Geometry check sheet. Reference: the model listing, model coordinates, mm. Coordinates: 2 decimals unless noted, no trailing zeros. Write each loop counter-clockwise with the first axis right and the second up, starting at its lowest first coordinate (ties: lowest second). Pieces come first, ordered by that corner, then holes. Notation, with made-up numbers: (73.25, -14) -> (91.25, -14) arc R18 cw to (91.25, 13) -> close; hole circle Ø4 at (82.25, 38). An arc over 180 degrees is marked (long way). Put each result on its own line as item: value. Start each with the question number.
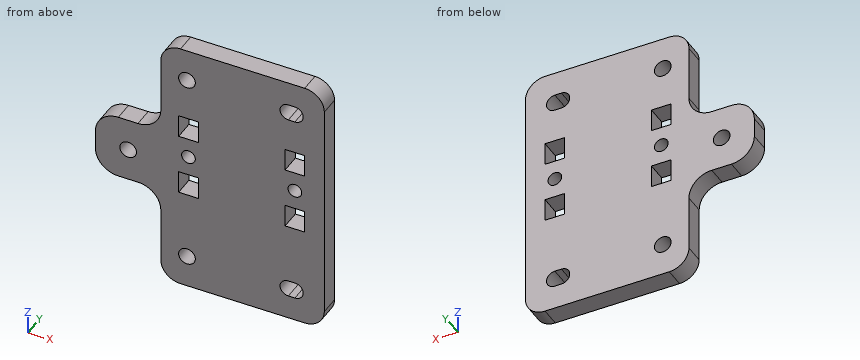
from build123d import *

# Parameters (mm, degrees)
SKETCH_1_R           = 2.55
EXTRUDE_1_DEPTH      = 6
SKETCH_2_R           = 2.55
CUT_EXTRUDE_1_DEPTH  = 7
SKETCH_3_R           = 2.1
SKETCH_3_W           = 7
SKETCH_3_H           = 6
CUT_EXTRUDE_11_DEPTH = 7
SKETCH_31_R          = 2.1
SKETCH_31_W          = 7
SKETCH_31_H          = 6
CUT_EXTRUDE_12_DEPTH = 7


with BuildPart() as part:
    # Эскиз1 → Бобышка-Вытянуть1 (new body)
    with BuildSketch(Plane(origin=(0, 0, 0), x_dir=(1, 0, 0), z_dir=(0, 1, 0))):
        with BuildLine():
            Line((-32, -10), (-38, -10))
            ThreePointArc((-38, -10), (-42.949747468, -7.949747468), (-45, -3))
            Line((-45, -3), (-45, 3))
            ThreePointArc((-45, 3), (-42.949747468, 7.949747468), (-38, 10))
            Line((-38, 10), (-32, 10))
            ThreePointArc((-32, 10), (-27.050252532, 12.050252532), (-25, 17))
            Line((-25, 17), (-25, 34))
            ThreePointArc((-25, 34), (-23.242640687, 38.242640687), (-19, 40))
            Line((-19, 40), (19, 40))
            ThreePointArc((19, 40), (23.242640687, 38.242640687), (25, 34))
            Line((25, 34), (25, -34))
            ThreePointArc((25, -34), (23.242640687, -38.242640687), (19, -40))
            Line((19, -40), (-19, -40))
            ThreePointArc((-19, -40), (-23.242640687, -38.242640687), (-25, -34))
            Line((-25, -34), (-25, -17))
            ThreePointArc((-25, -17), (-27.050252532, -12.050252532), (-32, -10))
        make_face()
        with Locations((-35, 0)):
            Circle(SKETCH_1_R, mode=Mode.SUBTRACT)
    extrude(amount=EXTRUDE_1_DEPTH)

    # Эскиз2 → Вырез-Вытянуть1 (cut, through all)
    with BuildSketch(Plane.XZ):
        with Locations((-17, -30)):
            Circle(SKETCH_2_R)
        with Locations((-17, 30)):
            Circle(SKETCH_2_R)
        with BuildLine():
            Line((16, -32.55), (14, -32.55))
            ThreePointArc((14, -32.55), (11.45, -30), (14, -27.45))
            Line((14, -27.45), (16, -27.45))
            ThreePointArc((16, -27.45), (18.55, -30), (16, -32.55))
        make_face()
        with BuildLine():
            Line((16, 32.55), (14, 32.55))
            ThreePointArc((14, 32.55), (11.45, 30), (14, 27.45))
            Line((14, 27.45), (16, 27.45))
            ThreePointArc((16, 27.45), (18.55, 30), (16, 32.55))
        make_face()
    extrude(amount=-CUT_EXTRUDE_1_DEPTH, mode=Mode.SUBTRACT)

    # Эскиз3 → Вырез-Вытянуть11 (cut, through all)
    with BuildSketch(Plane(origin=(-31, 0, 4), x_dir=(0, 0, -1), z_dir=(0, -1, 0))):
        with Locations((0, 47)):
            Circle(SKETCH_3_R)
        with Locations((9.531849908, 47)):
            Rectangle(SKETCH_3_W, SKETCH_3_H)
        with Locations((-9.531849908, 47)):
            Rectangle(SKETCH_3_W, SKETCH_3_H)
    extrude(amount=-CUT_EXTRUDE_11_DEPTH, mode=Mode.SUBTRACT)

    # Эскиз31 → Вырез-Вытянуть12 (cut, through all)
    with BuildSketch(Plane(origin=(30.45, 0, 4), x_dir=(0, 0, 1), z_dir=(0, -1, 0))):
        with Locations((0, 47)):
            Circle(SKETCH_31_R)
        with Locations((9.531849908, 47)):
            Rectangle(SKETCH_31_W, SKETCH_31_H)
        with Locations((-9.531849908, 47)):
            Rectangle(SKETCH_31_W, SKETCH_31_H)
    extrude(amount=-CUT_EXTRUDE_12_DEPTH, mode=Mode.SUBTRACT)


solid = part.part
Item 1: Go/stop test with flat-tipped pins: P1, Ø3, axis at y = 2.5, z = 18.5, coming from the -X side; P2, Ø3, axis at y = 3.5, z = -5, coming from the -X side; P3, Ø1.5, axis at y = 4, z = 12, coming from the -X side. Record where each tip stops, or that it passes through.
Item 2: Section check B-B, the plane z = 30. Enter the section's corners in (x, y), and give its area (3 significant figures).
Item 3: Section check C-C, the plane z = 0. Enter the section's corners in (x, y).
Item 4: Section check D-D, the plane x = -16.55. Enter the section's corners in (y, z), and give its area (3 significant figures).
Item 5: Scan lines: line 1 along X through (y, z) = (2.55, 4); line 2 along Z through (x, y) = (15.5, 2.05); line 3 along Z through (x, y) = (-19, 3.4). Record each from-to range of solid material in increasing order. Write a range as [from, to].
Item 6: Section check A-A, the plane x = -35. Enter the section's corners in (y, z), and give its area (3 significant figures).
From the geometry:
1. P1: x = -25
1. P2: x = -44.98
1. P3: x = -28.01
2. outline: (-25, 0) -> (-19.55, 0) -> (-19.55, 6) -> (-25, 6) -> close; (-14.45, 0) -> (11.45, 0) -> (11.45, 6) -> (-14.45, 6) -> close; (18.55, 0) -> (25, 0) -> (25, 6) -> (18.55, 6) -> close
2. area: 227 mm²
3. outline: (-45, 0) -> (-37.55, 0) -> (-37.55, 6) -> (-45, 6) -> close; (-32.45, 0) -> (25, 0) -> (25, 6) -> (-32.45, 6) -> close
4. outline: (0, -40) -> (6, -40) -> (6, -32.51) -> (0, -32.51) -> close; (0, -27.49) -> (6, -27.49) -> (6, -9.03) -> (0, -9.03) -> close; (0, -2.03) -> (6, -2.03) -> (6, 1.9) -> (0, 1.9) -> close; (0, 6.1) -> (6, 6.1) -> (6, 10.03) -> (0, 10.03) -> close; (0, 17.03) -> (6, 17.03) -> (6, 27.49) -> (0, 27.49) -> close; (0, 32.51) -> (6, 32.51) -> (6, 40) -> (0, 40) -> close
4. area: 311 mm²
5. line 1: [-44.93, -18.65], [-14.45, 13.9], [18.1, 25]
5. line 2: [-40, -32.55], [-27.45, -9.03], [-2.03, 1.96], [6.04, 10.03], [17.03, 27.45], [32.55, 40]
5. line 3: [-40, -31.58], [-28.42, -9.03], [-2.03, 10.03], [17.03, 28.42], [31.58, 40]
6. outline: (0, -10) -> (6, -10) -> (6, -2.55) -> (0, -2.55) -> close; (0, 2.55) -> (6, 2.55) -> (6, 10) -> (0, 10) -> close
6. area: 89.4 mm²
